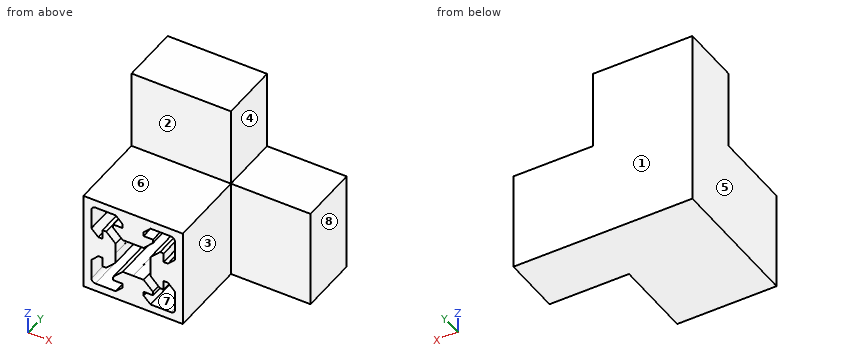
from build123d import *

# Parameters (mm, degrees)
BOSS_EXTRUDE1_DEPTH      = 15
BOSS_EXTRUDE1_DEPTH_BACK = 20
SKETCH3_W                = 25
SKETCH3_H                = 25
CUT_EXTRUDE1_DEPTH       = 30
SKETCH5_W                = 25
SKETCH5_H                = 15
BOSS_EXTRUDE2_DEPTH      = 20
SKETCH6_W                = 25
SKETCH6_H                = 15
BOSS_EXTRUDE3_DEPTH      = 20


with BuildPart() as part:
    # Sketch3 → Boss-Extrude1 (new, two sides: drawn at the far end of the back side and taken through both)
    with BuildSketch(Plane(origin=(0, 0, 0), x_dir=(1, 0, 0), z_dir=(0, 1, 0)).offset(-BOSS_EXTRUDE1_DEPTH_BACK)):
        Rectangle(SKETCH3_W, SKETCH3_H)
    extrude(amount=BOSS_EXTRUDE1_DEPTH + BOSS_EXTRUDE1_DEPTH_BACK)

    # Extrusion Profile → Cut-Extrude1 (cut)
    with BuildSketch(Plane(origin=(0, -20, 0), x_dir=(-1, 0, 0), z_dir=(0, -1, 0))):
        with BuildLine():
            Line((4.4, -0.002893219), (4.397106781, 0))
            Line((4.397106781, 0), (4.4, 0.002893219))
            Line((4.4, 0.002893219), (4.4, 2.632233047))
            Line((4.4, 2.632233047), (6.767766953, 5))
            Line((6.767766953, 5), (7.7, 5))
            Line((7.7, 5), (7.7, 2.625))
            Line((7.7, 2.625), (8.752106781, 2.625))
            Line((8.752106781, 2.625), (10.5, 4.372893219))
            Line((10.5, 4.372893219), (10.5, 9.5))
            ThreePointArc((10.5, 9.5), (10.207106781, 10.207106781), (9.5, 10.5))
            Line((9.5, 10.5), (4.372893219, 10.5))
            Line((4.372893219, 10.5), (2.625, 8.752106781))
            Line((2.625, 8.752106781), (2.625, 7.7))
            Line((2.625, 7.7), (5, 7.7))
            Line((5, 7.7), (5, 6.767766953))
            Line((5, 6.767766953), (2.632233047, 4.4))
            Line((2.632233047, 4.4), (0.002893219, 4.4))
            Line((0.002893219, 4.4), (0, 4.397106781))
            Line((0, 4.397106781), (-0.002893219, 4.4))
            Line((-0.002893219, 4.4), (-2.632233047, 4.4))
            Line((-2.632233047, 4.4), (-5, 6.767766953))
            Line((-5, 6.767766953), (-5, 7.7))
            Line((-5, 7.7), (-2.625, 7.7))
            Line((-2.625, 7.7), (-2.625, 8.752106781))
            Line((-2.625, 8.752106781), (-4.372893219, 10.5))
            Line((-4.372893219, 10.5), (-9.5, 10.5))
            ThreePointArc((-9.5, 10.5), (-10.207106781, 10.207106781), (-10.5, 9.5))
            Line((-10.5, 9.5), (-10.5, 4.372893219))
            Line((-10.5, 4.372893219), (-8.752106781, 2.625))
            Line((-8.752106781, 2.625), (-7.7, 2.625))
            Line((-7.7, 2.625), (-7.7, 5))
            Line((-7.7, 5), (-6.767766953, 5))
            Line((-6.767766953, 5), (-4.4, 2.632233047))
            Line((-4.4, 2.632233047), (-4.4, 0.002893219))
            Line((-4.4, 0.002893219), (-4.397106781, 0))
            Line((-4.397106781, 0), (-4.4, -0.002893219))
            Line((-4.4, -0.002893219), (-4.4, -2.632233047))
            Line((-4.4, -2.632233047), (-6.767766953, -5))
            Line((-6.767766953, -5), (-7.7, -5))
            Line((-7.7, -5), (-7.7, -2.625))
            Line((-7.7, -2.625), (-8.752106781, -2.625))
            Line((-8.752106781, -2.625), (-10.5, -4.372893219))
            Line((-10.5, -4.372893219), (-10.5, -9.5))
            ThreePointArc((-10.5, -9.5), (-10.207106781, -10.207106781), (-9.5, -10.5))
            Line((-9.5, -10.5), (-4.372893219, -10.5))
            Line((-4.372893219, -10.5), (-2.625, -8.752106781))
            Line((-2.625, -8.752106781), (-2.625, -7.7))
            Line((-2.625, -7.7), (-5, -7.7))
            Line((-5, -7.7), (-5, -6.767766953))
            Line((-5, -6.767766953), (-2.632233047, -4.4))
            Line((-2.632233047, -4.4), (-0.002893219, -4.4))
            Line((-0.002893219, -4.4), (0, -4.397106781))
            Line((0, -4.397106781), (0.002893219, -4.4))
            Line((0.002893219, -4.4), (2.632233047, -4.4))
            Line((2.632233047, -4.4), (5, -6.767766953))
            Line((5, -6.767766953), (5, -7.7))
            Line((5, -7.7), (2.625, -7.7))
            Line((2.625, -7.7), (2.625, -8.752106781))
            Line((2.625, -8.752106781), (4.372893219, -10.5))
            Line((4.372893219, -10.5), (9.5, -10.5))
            ThreePointArc((9.5, -10.5), (10.207106781, -10.207106781), (10.5, -9.5))
            Line((10.5, -9.5), (10.5, -4.372893219))
            Line((10.5, -4.372893219), (8.752106781, -2.625))
            Line((8.752106781, -2.625), (7.7, -2.625))
            Line((7.7, -2.625), (7.7, -5))
            Line((7.7, -5), (6.767766953, -5))
            Line((6.767766953, -5), (4.4, -2.632233047))
            Line((4.4, -2.632233047), (4.4, -0.002893219))
        make_face()
    extrude(amount=-CUT_EXTRUDE1_DEPTH, mode=Mode.SUBTRACT)

    # Sketch5 → Boss-Extrude2 (add)
    with BuildSketch(Plane.XY.offset(12.5)):
        with Locations((0, 7.5)):
            Rectangle(SKETCH5_W, SKETCH5_H)
    extrude(amount=BOSS_EXTRUDE2_DEPTH)

    # Sketch6 → Boss-Extrude3 (add)
    with BuildSketch(Plane(origin=(12.5, 0, 0), x_dir=(0, 0, -1), z_dir=(1, 0, 0))):
        with Locations((0, 7.5)):
            Rectangle(SKETCH6_W, SKETCH6_H)
    extrude(amount=BOSS_EXTRUDE3_DEPTH)


solid = part.part
CAD build for the part. Positions are in the model's coordinates, mm. Face numbers are marked on the shaded views. A direction names the side the tool comes from. Give positions to 0.01 mm unless a question says otherwise; leave off trailing zeros. Write each loop counter-clockwise with the first axis right and the second up, starting at its lowest first coordinate (ties: lowest second). Pieces come first, ordered by that corner, then holes. Notation, with made-up numbers: M 8.25,85.25 L 32.25,85.25 A30 ccw 32.25,118.25 Z; hole C 21.5,89.25 d5. An arc over 180 degrees is marked long. Put each result on its own line as item: value. Start each with the question number.
(1) Mould opens along X. For the marked faces 5, 6, 7 and 8 say: +X half, -X half, draft (parallel to the pull), parting line (faces both ways), or undercut.
(2) Band-saw the part on C-C, the plane x = 19.5. Write the cut outline in (y, z), and give its area (3 significant figures).
(3) Band-saw the part on B-B, the plane z = 20. Write the cut outline in (x, y), and give its area (3 significant figures).
(4) Which spindle directions (+Z, -Z, +X, -X, +Y, -Y) get a long thin tool onto all of the face, cutting with end or side? Do the marked faces 1, 2, 3 and 4. Say none if no direction does.
(5) Flat gauge pins, fed straight in: pin 1 Ø1 at (x, y) = (-7.5, -10) entering from +Z; pin 2 Ø8 at (y, z) = (6, 15.5) entering from +X; pin 3 Ø2 at (y, z) = (-7.5, -1) entering from +X; pin 4 Ø10 at (x, z) = (18, 2) entering from -Y. Where does each tip first touch, or does it go through?
(6) Band-saw the part on A-A, the plane x = 2. Write the cut outline in (y, z), and give its area (3 significant figures).
(7) Probe L1, parallel to Z at x = 8, y = 8 (3 decimals); L2, parallel to X at y = 3.5, z = -7; L3, parallel to X at y = -0.5, z = 4.5. List the from-to ranges inside material, lowest first.
Response values:
1. face 5: -X half
1. face 6: draft
1. face 7: undercut
1. face 8: +X half
2. outline: M 0,-12.5 L 15,-12.5 L 15,12.5 L 0,12.5 Z
2. area: 375 mm2
3. outline: M -12.5,0 L 12.5,0 L 12.5,15 L -12.5,15 Z
3. area: 375 mm2
4. face 1: +Z, -Z, +X, -X, +Y
4. face 2: +Z, +X, -X, -Y
4. face 3: +Z, -Z, +X, -Y
4. face 4: +Z, +X, +Y, -Y
5. pin 1: stops at z = 12.5
5. pin 2: stops at x = 32.5
5. pin 3: stops at x = 12.5
5. pin 4: stops at y = 0
6. outline: M -20,-12.5 L 15,-12.5 L 15,32.5 L 0,32.5 L 0,12.5 L -20,12.5 L -20,4.4 L 10,4.4 L 10,-4.4 L -20,-4.4 Z
6. area: 911 mm2
7. L1: z = -12.5 to -10.5, -2.625 to 2.625, 10.5 to 32.5
7. L2: x = -12.5 to -10.5, -5 to 5, 10.5 to 32.5
7. L3: x = -12.5 to -10.5, -7.7 to -6.27, -2.73 to 2.73, 6.27 to 7.7, 10.5 to 12.5
